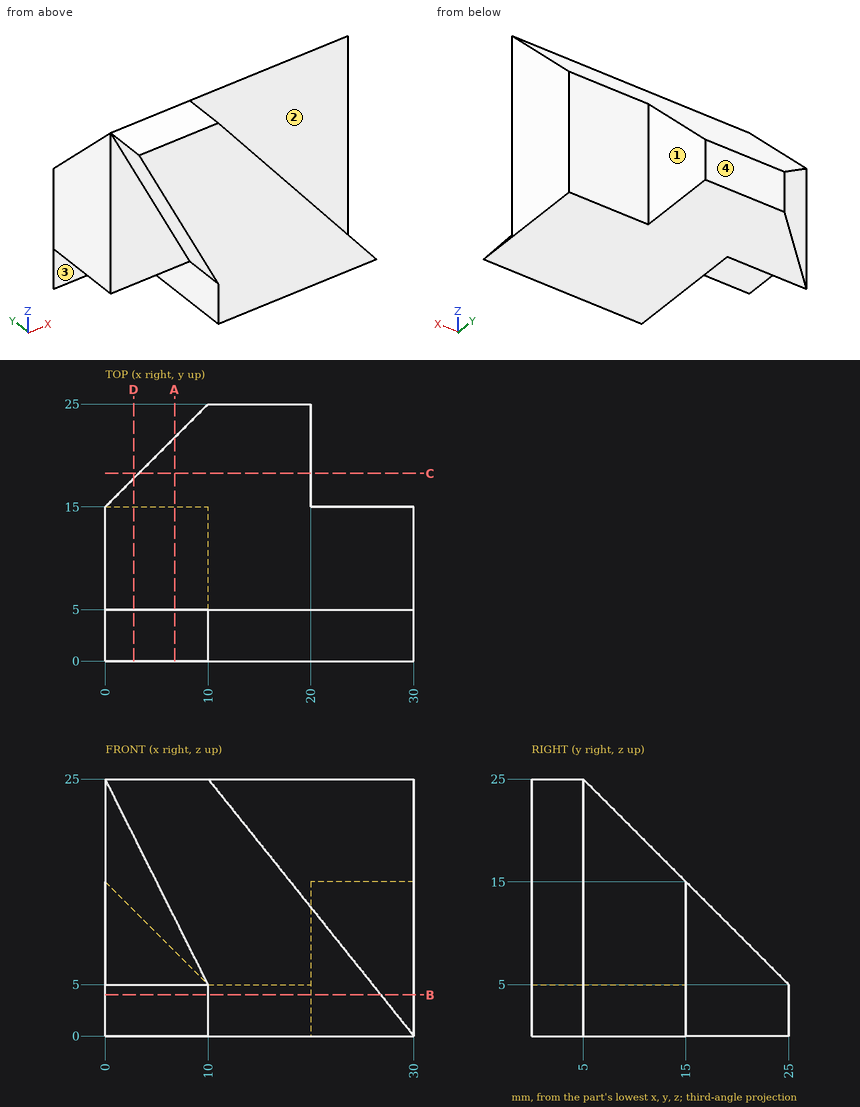
Geometry check sheet. Reference: drawing and pictorial views, mm from the part's lowest x, y, z. A direction names the side the tool comes from. Round coordinates to 2 decimals unless told otherwise and drop trailing zeros. Order: outer loops, then holes, each group sorted by start corner. A loop starts at its lowest first (then second) coordinate and runs counter-clockwise, first axis right, second up. Notation, with made-up numbers: M 0.5,21 L 17.5,21 A12 ccw 17.5,25 Z; hole C 45.25,51.5 d1. An arc over 180 degrees is marked long. Answer as CSV lines item,"result".
1) Sectioned sample at B-B on z = 4. Record the cut outline in (x, y), and give its area (3 significant figures).
Entries:
outline,"M 0,15 L 10,15 L 10,0 L 26.8,0 L 26.8,5 L 30,5 L 30,15 L 20,15 L 20,25 L 10,25 Z"
area,"434 mm2"
2) Thickness scan on probe 1 along Y at (x, z) = (25.75, 10.75); probe 2 along X at (y, z) = (5.75, 2); probe 3 along Y at (x, z) = (1.75, 11.5). Record the ranges inside material, lowest first. Write a range as [from, to].
Entries:
probe 1,"[5, 15]"
probe 2,"[10, 30]"
probe 3,"[5, 16.75]"
3) Tool access check on the marked faces 1, 2, 3 and 4. Record the directions out of +Z, -Z, +X, -X, +Y, -Y that give a thin tool (end or side, any length) a straight path to the whole face; none if there is none.
Entries:
face 1,"+Z, -Z, +X, +Y"
face 2,"+Z, +X, -Y"
face 3,"-Z, -X, -Y"
face 4,"+Z, -Z, +X, -X, +Y"
4) Sectioned sample at A-A on x = 6.75. Record the cut outline in (y, z), and give its area (3 significant figures).
Entries:
outline,"M 0,11.5 L 5,11.5 L 5,5 L 15,5 L 15,0 L 21.75,0 L 21.75,8.25 L 5,25 L 0,25 Z"
area,"296 mm2"
5) Sectioned sample at D-D on x = 2.75. Record the cut outline in (y, z), and give its area (3 significant figures).
Entries:
outline,"M 0,19.5 L 5,19.5 L 5,5 L 15,5 L 15,0 L 17.75,0 L 17.75,12.25 L 5,25 L 0,25 Z"
area,"215 mm2"
6) Gauge pin test, flat ends, axial feed: pin 1 Ø6 at (x, z) = (20, 14) entering from -Y; pin 2 Ø3 at (y, z) = (18.5, 7.5) entering from +X; pin 3 Ø1.5 at (x, z) = (9.5, 7) entering from +Y; pin 4 Ø2.5 at (y, z) = (6.5, 3.5) entering from -X. Record the tip position at first contact, or that the pin passes through.
Entries:
pin 1,"y = 0"
pin 2,"x = 20"
pin 3,"y = 23.75"
pin 4,"x = 10"
7) Sectioned sample at C-C on y = 18.25. Record the cut outline in (x, z).
Entries:
outline,"M 3.25,0 L 20,0 L 20,11.75 L 3.25,11.75 Z"
